```python
from build123d import *

# Parameters (mm, degrees)
SKETCH1_W           = 14
SKETCH1_H           = 14
BOSS_EXTRUDE1_DEPTH = 1.6
CUT_EXTRUDE1_DEPTH  = 96.918055802
FILLET1_R           = 3


with BuildPart() as part:
    # Sketch1 → Boss-Extrude1 (new body)
    with BuildSketch(Plane.XY):
        with BuildLine():
            Line((-78.750976664, 0.641871894), (-78.750976664, 47.553166294))
            ThreePointArc((-78.750976664, 47.553166294), (-77.871635054, 49.67514838), (-75.749104672, 50.553165702))
            Line((-75.749104672, 50.553165702), (78.500895328, 50.456909802))
            ThreePointArc((78.500895328, 50.456909802), (80.621005422, 49.577568802), (81.499023352, 47.456910433))
            Line((81.499023352, 47.456910433), (81.499023352, -24.544961067))
            ThreePointArc((81.499023352, -24.544961067), (80.620343696, -26.666281411), (78.499023352, -27.544961067))
            Line((78.499023352, -27.544961067), (19.649835152, -27.544961067))
            ThreePointArc((19.649835152, -27.544961067), (19.499213793, -27.548744585), (19.348972354, -27.560085596))
            Line((19.348972354, -27.560085596), (-18.050925646, -31.329836596))
            ThreePointArc((-18.050925646, -31.329836596), (-18.201167086, -31.341177607), (-18.351788445, -31.344961125))
            Line((-18.351788445, -31.344961125), (-66.088698945, -31.344961125))
            ThreePointArc((-66.088698945, -31.344961125), (-67.842829771, -30.778687705), (-68.934748827, -29.2936445))
            Line((-68.934748827, -29.2936445), (-78.597026527, -0.3068115))
            ThreePointArc((-78.597026527, -0.3068115), (-78.712239029, 0.161325115), (-78.750976664, 0.641871894))
        make_face()
        with Locations((67.999023336, -17.044961106)):
            Rectangle(SKETCH1_W, SKETCH1_H, mode=Mode.SUBTRACT)
        with Locations((-46.000976664, 1.955038894)):
            Rectangle(SKETCH1_W, SKETCH1_H, mode=Mode.SUBTRACT)
        with Locations((-43.000976664, 39.955038894)):
            Rectangle(SKETCH1_W, SKETCH1_H, mode=Mode.SUBTRACT)
        with Locations((-24.000976664, 39.955038894)):
            Rectangle(SKETCH1_W, SKETCH1_H, mode=Mode.SUBTRACT)
        with Locations((-5.000976664, 39.955038894)):
            Rectangle(SKETCH1_W, SKETCH1_H, mode=Mode.SUBTRACT)
        with Locations((13.999023336, 39.955038894)):
            Rectangle(SKETCH1_W, SKETCH1_H, mode=Mode.SUBTRACT)
        with Locations((32.999023336, 39.955038894)):
            Rectangle(SKETCH1_W, SKETCH1_H, mode=Mode.SUBTRACT)
        with Locations((51.999023336, 39.955038894)):
            Rectangle(SKETCH1_W, SKETCH1_H, mode=Mode.SUBTRACT)
        with Locations((70.999023336, 39.955038894)):
            Rectangle(SKETCH1_W, SKETCH1_H, mode=Mode.SUBTRACT)
        with Locations((-35.970976664, 20.955038894)):
            Rectangle(SKETCH1_W, SKETCH1_H, mode=Mode.SUBTRACT)
        with Locations((-16.970976664, 20.955038894)):
            Rectangle(SKETCH1_W, SKETCH1_H, mode=Mode.SUBTRACT)
        with Locations((2.029023336, 20.955038894)):
            Rectangle(SKETCH1_W, SKETCH1_H, mode=Mode.SUBTRACT)
        with Locations((21.029023336, 20.955038894)):
            Rectangle(SKETCH1_W, SKETCH1_H, mode=Mode.SUBTRACT)
        with Locations((40.029023336, 20.955038894)):
            Rectangle(SKETCH1_W, SKETCH1_H, mode=Mode.SUBTRACT)
        with Locations((63.779023336, 20.955038894)):
            Rectangle(SKETCH1_W, SKETCH1_H, mode=Mode.SUBTRACT)
        with Locations((-27.000976664, 1.955038894)):
            Rectangle(SKETCH1_W, SKETCH1_H, mode=Mode.SUBTRACT)
        with Locations((-8.000976664, 1.955038894)):
            Rectangle(SKETCH1_W, SKETCH1_H, mode=Mode.SUBTRACT)
        with Locations((10.999023336, 1.955038894)):
            Rectangle(SKETCH1_W, SKETCH1_H, mode=Mode.SUBTRACT)
        with Locations((29.999023336, 1.955038894)):
            Rectangle(SKETCH1_W, SKETCH1_H, mode=Mode.SUBTRACT)
        with Locations((48.999023336, 1.955038894)):
            Rectangle(SKETCH1_W, SKETCH1_H, mode=Mode.SUBTRACT)
        with Locations((67.999023336, 1.955038894)):
            Rectangle(SKETCH1_W, SKETCH1_H, mode=Mode.SUBTRACT)
        with Locations((29.999023336, -17.044961106)):
            Rectangle(SKETCH1_W, SKETCH1_H, mode=Mode.SUBTRACT)
        with Locations((48.999023336, -17.044961106)):
            Rectangle(SKETCH1_W, SKETCH1_H, mode=Mode.SUBTRACT)
        with Locations((-53.000976664, -20.844961106)):
            Rectangle(SKETCH1_W, SKETCH1_H, mode=Mode.SUBTRACT)
        with Locations((-24.500976664, -20.844961106)):
            Rectangle(SKETCH1_W, SKETCH1_H, mode=Mode.SUBTRACT)
    extrude(amount=BOSS_EXTRUDE1_DEPTH)

    # Sketch2 → Cut-Extrude1 (cut, through all)
    with BuildSketch(Plane.XY.offset(1.6)):
        Polygon((-52.113994262, 52.196412896), (-52.113994262, 11.585140269), (-55.415723743, 11.585140269), (-55.415723743, -10.206274311), (-62.184269181, -10.206274311), (-62.184269181, -38.601147855), (-84.470943183, -34.143813054), (-95.201563999, 49.885202259), (-53.764859002, 58.304612437), align=None)
    extrude(amount=-CUT_EXTRUDE1_DEPTH, mode=Mode.SUBTRACT)

    # Fillet1
    fillet1_edges = [part.edges().sort_by_distance(p)[0] for p in [
        (-52.113994262, 50.538416795, 0.8),
        (-62.184269181, -31.344961125, 0.8),
        (-62.184269181, -10.206274311, 0.8),
        (-55.415723743, 11.585140269, 0.8),
    ]]
    fillet(fillet1_edges, radius=FILLET1_R)


solid = part.part
```
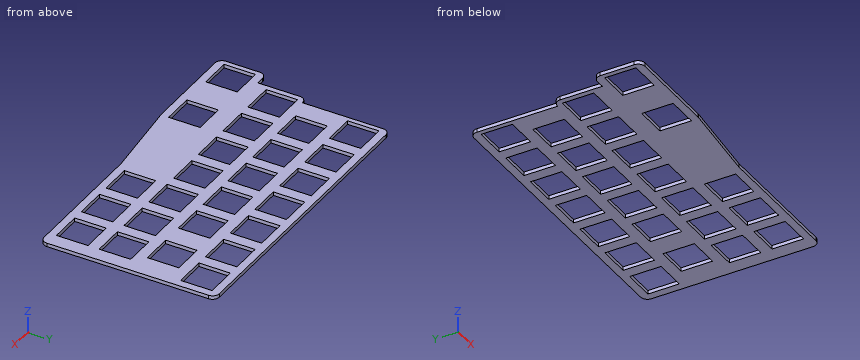
Geometry: final body of the model. Coordinates: model frame, mm. Round coordinates to 2 decimals unless told otherwise and drop trailing zeros. Write each loop counter-clockwise with the first axis right and the second up, starting at its lowest first coordinate (ties: lowest second). Pieces come first, ordered by that corner, then holes.
Item 1: Section query A-A (y = -3.5). Give the number of separate pieces and of enclosed holes in the cut face, plus the area to 3 significant figures.
Item 2: Section query B-B (y = 22.5). Return loops of the section in (x, z), plus the area to 3 significant figures.
Item 3: Pin query (flat end, axial travel): P1, Ø0.5, axis at y = 39.5, z = 1, coming from the -X side; P2, Ø0.5, axis at x = 66, z = 1, coming from the +Y side. Return the tip coordinate at first contact, or that it passes through.
Item 4: Material intervals for L1, parallel to Y at x = 36, z = 0.7; L2, parallel to Y at x = -38, z = 0.7; L3, parallel to Y at x = 32, z = 0.55, sorted ascending.
Completed:
1. separate pieces: 8
1. enclosed holes: 0
1. area: 62.3 mm2
2. outline: (-52.11, 0) - (-42.97, 0) - (-42.97, 1.6) - (-52.11, 1.6) - close; (-28.97, 0) - (-23.97, 0) - (-23.97, 1.6) - (-28.97, 1.6) - close; (-9.97, 0) - (-4.97, 0) - (-4.97, 1.6) - (-9.97, 1.6) - close; (9.03, 0) - (14.03, 0) - (14.03, 1.6) - (9.03, 1.6) - close; (28.03, 0) - (33.03, 0) - (33.03, 1.6) - (28.03, 1.6) - close; (47.03, 0) - (56.78, 0) - (56.78, 1.6) - (47.03, 1.6) - close; (70.78, 0) - (81.5, 0) - (81.5, 1.6) - (70.78, 1.6) - close
2. area: 79.4 mm2
3. P1: stops at x = -52.11
3. P2: stops at y = 50.46
4. L1: y = -27.54 to -24.04, -10.04 to -5.04, 8.96 to 13.96, 27.96 to 32.96, 46.96 to 50.48
4. L2: y = -31.34 to 13.96, 27.96 to 32.96, 46.96 to 50.53
4. L3: y = -27.54 to -24.04, -10.04 to -5.04, 8.96 to 32.96, 46.96 to 50.49
